Part print with two shaded views. Sizes in mm from the minimum x, y, z corner. Give positions to 0.01 mm unless a question says otherwise; leave off trailing zeros. Order: outer loops, then holes, each group sorted by start corner. A loop starts at its lowest first (then second) coordinate and runs counter-clockwise, first axis right, second up. Notation, with made-up numbers: M 87.5,62.25 L 124.5,62.25 A16 cw 124.5,92.25 Z; hole C 11,-33.5 d6. An arc over 180 degrees is marked long. Write each question's results on one line, items separated by ' | '. Start each with the question number.
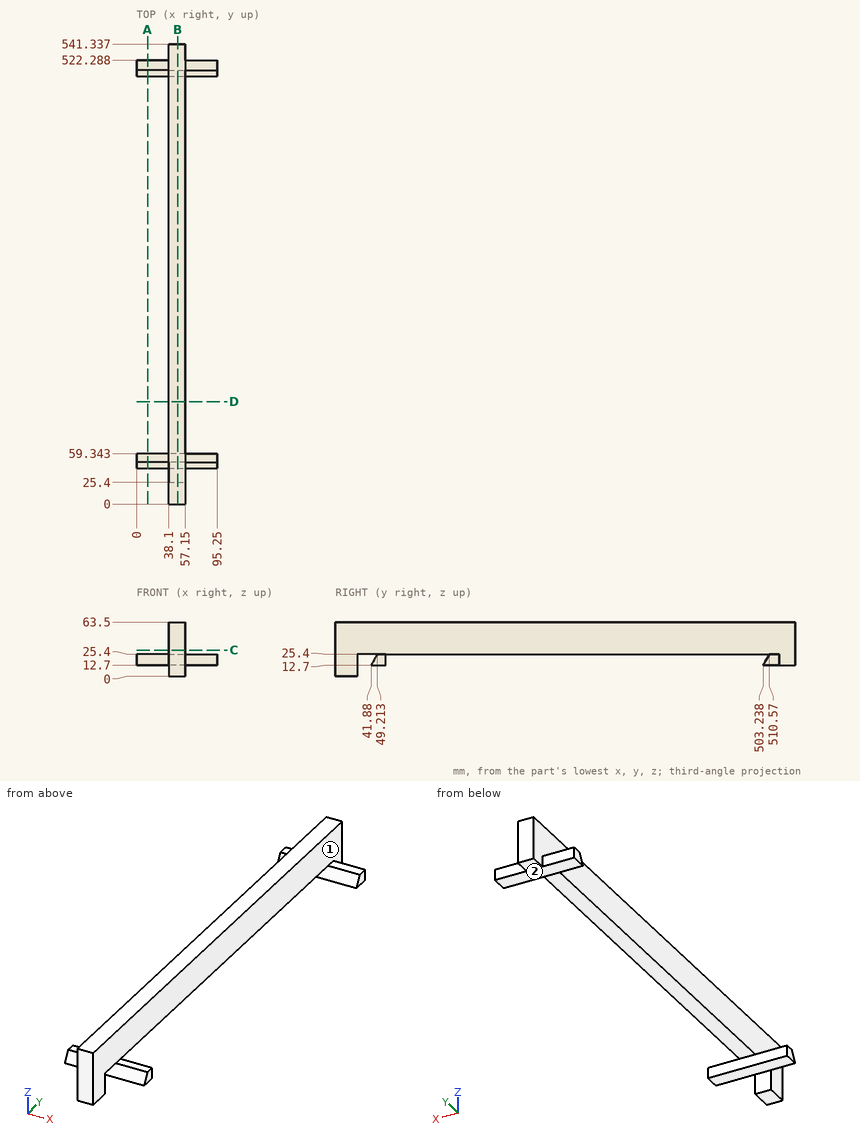
(1) Probe L1, parallel to Z at x = 47, y = 464; L2, parallel to X at y = 429.5, z = 41.5; L3, parallel to Y at x = 54, z = 23.5 (1 decimal). List the from-to ranges inside material, lowest first.
(2) Drop flat-ended pins along their axis: P1, Ø5, axis at x = 79, y = 52.5, coming from the +Z side; P2, Ø1, axis at y = 484.5, z = 51.5, coming from the -X side; P3, Ø1, axis at x = 49, y = 439, coming from the -Z side. Give the stop position or say it passes through.
(3) Saw through at C-C on z = 30.5. Give the cut face in (x, y).
(4) Pull direction Z, two halves, no side cores. Call the marked faces 1 and 2: +Z half, -Z half, draft (parallel to the pull), parting line (faces both ways), or undercut.
(5) Saw through at B-B on x = 48.5. Give the cut face in (y, z), plus the area to 3 significant figures.
(6) Saw through at A-A on x = 13. Give the cut face in (y, z).
(7) Saw through at D-D on y = 120.5. Give the cut face in (x, z).
Taken from the geometry:
1) L1: z = 25.4 to 63.5 | L2: x = 38.1 to 57.15 | L3: y = 0 to 25.4, 48.1 to 59.3, 509.5 to 541.3
2) P1: stops at z = 25.4 | P2: stops at x = 38.1 | P3: stops at z = 25.4
3) outline: M 38.1,0 L 57.15,0 L 57.15,541.34 L 38.1,541.34 Z
4) face 1: draft | face 2: -Z half
5) outline: M 0,0 L 25.4,0 L 25.4,25.4 L 49.21,25.4 L 41.88,12.7 L 59.34,12.7 L 59.34,25.4 L 510.57,25.4 L 503.24,12.7 L 541.34,12.7 L 541.34,63.5 L 0,63.5 Z | area: 21,900 mm²
6) outline: M 41.88,12.7 L 59.34,12.7 L 59.34,25.4 L 49.21,25.4 Z; M 503.24,12.7 L 522.29,12.7 L 522.29,25.4 L 510.57,25.4 Z
7) outline: M 38.1,25.4 L 57.15,25.4 L 57.15,63.5 L 38.1,63.5 Z
